Here's how the part is built. I have some questions about the finished solid (model axes, mm). Round coordinates to 2 decimals unless told otherwise and drop trailing zeros. Loops run counter-clockwise (first coordinate to the right, second up) from the corner with the lowest first, then second, coordinate; pieces in that order, holes last. Notation, with made-up numbers: M -24,37.5 L 32,37.5 A36 cw 32,75.5 Z; hole C -20.5,-24.75 d1. An arc over 180 degrees is marked long. Use a Markdown table: item, result.
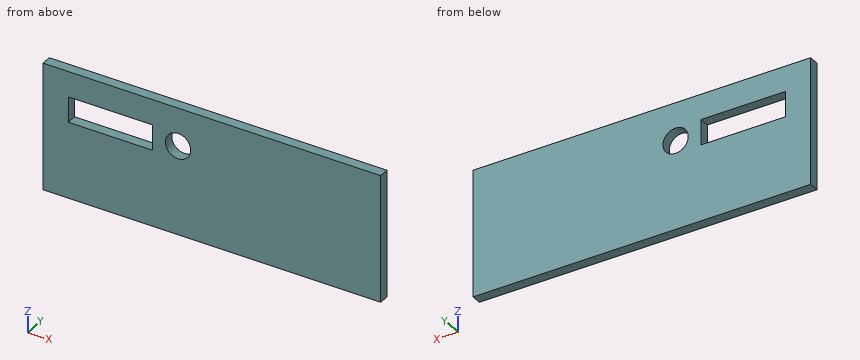
from build123d import *

# Parameters (mm, degrees)
SKETCH1_W           = 200
SKETCH1_H           = 75
BOSS_EXTRUDE1_DEPTH = 6
SKETCH2_R           = 7.5
SKETCH2_W           = 50
SKETCH2_H           = 15
CUT_EXTRUDE1_DEPTH  = 214.684346642


with BuildPart() as part:
    # Sketch1 → Boss-Extrude1 (new body)
    with BuildSketch(Plane(origin=(0, 0, 0), x_dir=(1, 0, 0), z_dir=(0, 1, 0))):
        with Locations((100, 37.5)):
            Rectangle(SKETCH1_W, SKETCH1_H)
    extrude(amount=BOSS_EXTRUDE1_DEPTH)

    # Sketch2 → Cut-Extrude1 (cut, through all)
    with BuildSketch(Plane(origin=(0, 6, 0), x_dir=(1, 0, 0), z_dir=(0, 1, 0))):
        with Locations(Location((80, 22.5, 0), (0, 0, 270))):
            Circle(SKETCH2_R)
        with Locations((40, 22.5)):
            Rectangle(SKETCH2_W, SKETCH2_H)
    extrude(amount=-CUT_EXTRUDE1_DEPTH, mode=Mode.SUBTRACT)


solid = part.part
1. Imagine slicing it at A-A, the plane z = -27. Write out the boundary of the cut face in (x, y).
Answer sheet:
| item | result |
|---|---|
| outline | M 0,0 L 15,0 L 15,6 L 0,6 Z; M 65,0 L 74,0 L 74,6 L 65,6 Z; M 86,0 L 200,0 L 200,6 L 86,6 Z |
2. Imagine slicing it at B-B, the plane y = 3.55. Write out the boundary of the cut face in (x, z).
Answer sheet:
| item | result |
|---|---|
| outline | M 0,-75 L 200,-75 L 200,0 L 0,0 Z; hole M 15,-30 L 65,-30 L 65,-15 L 15,-15 Z; hole C 80,-22.5 d15 |
3. Imagine slicing it at C-C, the plane x = 80. Write out the boundary of the cut face in (y, z).
Answer sheet:
| item | result |
|---|---|
| outline | M 0,-75 L 6,-75 L 6,-30 L 0,-30 Z; M 0,-15 L 6,-15 L 6,0 L 0,0 Z |
4. I need wall thicknesses on probe 1 along X at (y, z) = (4.5, -22.5); probe 2 along X at (y, z) = (4.1, -25.5); probe 3 along Z at (x, y) = (32, 3.95). Which ranges of each line are inside material? Lowest first, please. Write a range as from..to.
Answer sheet:
| item | result |
|---|---|
| probe 1 | 0..15, 65..72.5, 87.5..200 |
| probe 2 | 0..15, 65..73.13, 86.87..200 |
| probe 3 | -75..-30, -15..0 |
